```python
from build123d import *

# Parameters (mm, degrees)
SKETCH1_W           = 20.5
SKETCH1_H           = 24
BOSS_EXTRUDE1_DEPTH = 9
FILLET1_R           = 3
FILLET2_R           = 2
CUT_EXTRUDE1_REACH  = 47.453
SKETCH2_R           = 2
DRAFT1_START        = -1.394491884
DRAFT1_OUTLINE_W    = 64
DRAFT1_OUTLINE_H    = 35
DRAFT1_DEPTH        = 2.788983768


# Read off the part's stored shape, not the designer's step: Draft1
with BuildPart() as part:
    # Sketch1 → Boss-Extrude1 (new body)
    with BuildSketch(Plane(origin=(0, 0, 0), x_dir=(1, 0, 0), z_dir=(0, 1, 0))):
        Polygon((-26, 16), (26, 16), (26, -12), (31, -12), (31, -16), (26, -16), (-26, -16), (-31, -16), (-31, -12), (-26, -12), align=None)
        with Locations((-11.75, 0)):
            Rectangle(SKETCH1_W, SKETCH1_H, mode=Mode.SUBTRACT)
        with Locations((11.75, 0)):
            Rectangle(SKETCH1_W, SKETCH1_H, mode=Mode.SUBTRACT)
    extrude(amount=BOSS_EXTRUDE1_DEPTH)

    # Fillet1
    fillet1_edges = [part.edges().sort_by_distance(p)[0] for p in [
        (-1.5, 4.5, 12),
        (-1.5, 4.5, -12),
        (-22, 4.5, -12),
        (-22, 4.5, 12),
        (22, 4.5, 12),
        (22, 4.5, -12),
        (1.5, 4.5, -12),
        (1.5, 4.5, 12),
    ]]
    fillet(fillet1_edges, radius=FILLET1_R)

    # Fillet2
    fillet2_edges = [part.edges().sort_by_distance(p)[0] for p in [
        (-26, 4.5, -16),
        (26, 4.5, -16),
        (31, 4.5, 16),
        (31, 4.5, 12),
        (-31, 4.5, 12),
        (-31, 4.5, 16),
    ]]
    fillet(fillet2_edges, radius=FILLET2_R - 0.0001)  # a hair under: the kernel refuses the full size

    # Sketch2 → Cut-Extrude1 (cut, up to next)
    with BuildSketch(Plane(origin=(0, 0, -16), x_dir=(-1, 0, 0), z_dir=(0, 0, -1)), mode=Mode.PRIVATE) as cut_extrude1_sk1:
        with Locations((-13, 4.5)):
            Circle(SKETCH2_R)
    cut_extrude1_tool1 = extrude(cut_extrude1_sk1.sketch, amount=-CUT_EXTRUDE1_REACH, mode=Mode.PRIVATE) & part.part
    # Sketch2 → Cut-Extrude1 (cut, up to next)
    with BuildSketch(Plane(origin=(0, 0, -16), x_dir=(-1, 0, 0), z_dir=(0, 0, -1)), mode=Mode.PRIVATE) as cut_extrude1_sk2:
        with Locations(Location((13, 4.5, 0), (0, 0, 180))):
            Circle(SKETCH2_R)
    cut_extrude1_tool2 = extrude(cut_extrude1_sk2.sketch, amount=-CUT_EXTRUDE1_REACH, mode=Mode.PRIVATE) & part.part
    add(cut_extrude1_tool1.solids().sort_by_distance((13, 4.5, -16))[0], mode=Mode.SUBTRACT)
    add(cut_extrude1_tool2.solids().sort_by_distance((-13, 4.5, -16))[0], mode=Mode.SUBTRACT)

    # Draft1 outline → Draft1 (cut)
    with BuildSketch(Plane(origin=(0, 0, 0), x_dir=(1, 0, 0), z_dir=(0, 0.9961946980917455, -0.08715574274765824)).offset(DRAFT1_START)):
        with Locations((0, -0.5)):
            Rectangle(DRAFT1_OUTLINE_W, DRAFT1_OUTLINE_H)
    extrude(amount=DRAFT1_DEPTH, mode=Mode.SUBTRACT)


solid = part.part
```
CAD build for the part. Positions are in the model's coordinates, mm. A direction names the side the tool comes from. Give positions to 0.01 mm unless a question says otherwise; leave off trailing zeros. Order: outer loops, then holes, each group sorted by start corner. A loop starts at its lowest first (then second) coordinate and runs counter-clockwise, first axis right, second up. Notation, with made-up numbers: M -26.5,-2.5 L -17.5,-2.5 A16 ccw -17.5,27.5 Z; hole C -15.75,76 d9. An arc over 180 degrees is marked long. Put each result on its own line as item: value. Start each with the question number.
(1) Mould opens along X. For faces 1 (the cylindrical face through (-2.4, 4.74, -11.14)), 2 (the flat face through (0, 9, 1)), 3 (the flat face through (26, 6, -1)) say: +X half, -X half, draft (parallel to the pull), parting line (faces both ways), or undercut.
(2) Saw through at A-A, the plane z = -6. Write the cut outline in (x, y).
(3) Drill centre lines: line 1 along X through (y, z) = (1.75, -5.5); line 2 along Y through (x, z) = (-13, -14.1); line 3 along Z through (x, y) = (15, 3.75). Where is each one in solid material? Low to high.
(4) Saw through at B-B, the plane x = 13. Write the cut outline in (y, z), then the cut area to 3 significant figures.
(5) Which spindle directions (+Z, -Z, +X, -X, +Y, -Y) get a long thin tool onto all of the face, cutting with end or side? Do faces 4 (the cylindrical face through (2.36, 5.64, 11.1)), 5 (the flat face through (-26, 6, -1)), 6 (the cylindrical face through (25.4, 4.56, -15.43)), 7 (the cylindrical face through (14.6, 3.3, -14)), 8 (the cylindrical face through (-30.43, 5.86, 15.4)). Say none if no direction does.
(6) Flat gauge pins, fed straight in: pin 1 Ø2 at (y, z) = (3, 0.5) entering from -X; pin 2 Ø1 at (y, z) = (4.5, -1.5) entering from +X; pin 3 Ø3.5 at (x, y) = (28, 7) entering from -Z. Where does each tip first touch, or does it go through?
(7) Saw through at C-C, the plane x = -3. Write the cut outline in (y, z), then the cut area to 3 significant figures.
Check result:
1. face 1: undercut
1. face 2: draft
1. face 3: +X half
2. outline: M -26,0.87 L -22,0.87 L -22,9 L -26,9 Z; M -1.5,0.87 L 1.5,0.87 L 1.5,9 L -1.5,9 Z; M 22,0.87 L 26,0.87 L 26,9 L 22,9 Z
3. line 1: x = -26 to -22, -1.5 to 1.5, 22 to 26
3. line 2: y = 0.17 to 2.5, 6.5 to 9
3. line 3: z = -16 to -12, 12 to 16
4. outline: M 0,-16 L 2.5,-16 L 2.5,-12 L 0.35,-12 Z; M 2.45,12 L 9,12 L 9,16 L 2.8,16 Z; M 6.5,-16 L 9,-16 L 9,-12 L 6.5,-12 Z
4. area: 44.8 mm2
5. face 4: +Y, -Y
5. face 5: -Z, -X, +Y, -Y
5. face 6: -Z, +X, +Y, -Y
5. face 7: -Z
5. face 8: +Z, -X, +Y, -Y
6. pin 1: stops at x = -26
6. pin 2: stops at x = 26
6. pin 3: stops at z = 12
7. outline: M 0,-16 L 9,-16 L 9,-11.6 L 0.39,-11.6 Z; M 2.41,11.6 L 9,11.6 L 9,16 L 2.8,16 Z
7. area: 66.9 mm2
